For this review, take the finished solid that the model builds, in its own axes (mm). Round coordinates to 2 decimals unless told otherwise and drop trailing zeros. Order: outer loops, then holes, each group sorted by start corner. A loop starts at its lowest first (then second) coordinate and runs counter-clockwise, first axis right, second up. Notation, with made-up numbers: (74.25, 80) - (123.25, 80) arc R13 ccw to (123.25, 90) - close; hole circle Ø9 at (76, 50.5). An arc over 180 degrees is marked (long way). One line per question, with ' | ' between items.
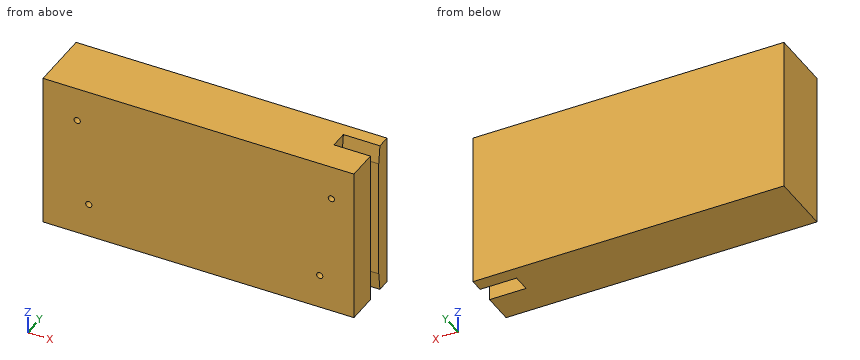
```python
from build123d import *

# Parameters (mm, degrees)
SCHIZZO2_W                   = 2000
SCHIZZO2_H                   = 1000
ESTRUSIONE_ESTRUSIONE1_DEPTH = 400
SVUOTA1_T                    = 40
SCHIZZO3_W                   = 320
SCHIZZO3_H                   = 545
ESTRUSIONE_ESTRUSIONE2_DEPTH = 285
SCHIZZO5_R                   = 20
TAGLIO_ESTRUSIONE1_DEPTH     = 40
SCHIZZO7_W                   = 235.156084519
SCHIZZO7_H                   = 1000
TAGLIO_ESTRUSIONE2_DEPTH     = 100
ESTRUSIONE_ESTRUSIONE4_DEPTH = 920
TAGLIO_ESTRUSIONE3_DEPTH     = 235.156084519


with BuildPart() as part:
    # Schizzo2 → Estrusione-Estrusione1 (new body)
    with BuildSketch(Plane(origin=(0, 0, 0), x_dir=(1, 0, 0), z_dir=(0, 1, 0))):
        Rectangle(SCHIZZO2_W, SCHIZZO2_H)
    extrude(amount=ESTRUSIONE_ESTRUSIONE1_DEPTH)

    # Svuota1 (no face opened: a closed hollow body)
    add(offset(amount=-SVUOTA1_T, mode=Mode.PRIVATE), mode=Mode.SUBTRACT)

    # Schizzo3 → Estrusione-Estrusione2 (add)
    with BuildSketch(Plane(origin=(0, 40, 0), x_dir=(1, 0, 0), z_dir=(0, 1, 0))):
        Rectangle(SCHIZZO3_W, SCHIZZO3_H)
    extrude(amount=ESTRUSIONE_ESTRUSIONE2_DEPTH)

    # Schizzo5 → Taglio-Estrusione1 (cut)
    with BuildSketch(Plane.XZ):
        with Locations(Location((-780, 280, 0), (0, 0, 270))):
            Circle(SCHIZZO5_R)
        with Locations(Location((780, -280, 0), (0, 0, 270))):
            Circle(SCHIZZO5_R)
        with Locations(Location((854.59, 280, 0), (0, 0, 270))):
            Circle(SCHIZZO5_R)
        with Locations(Location((-705.41, -280, 0), (0, 0, 270))):
            Circle(SCHIZZO5_R)
    extrude(amount=-TAGLIO_ESTRUSIONE1_DEPTH, mode=Mode.SUBTRACT)

    # Schizzo7 → Taglio-Estrusione2 (cut)
    with BuildSketch(Plane(origin=(0, 200, 0), x_dir=(1, 0, 0), z_dir=(0, 1, 0))):
        with Locations((882.421957741, 0)):
            Rectangle(SCHIZZO7_W, SCHIZZO7_H)
    extrude(amount=TAGLIO_ESTRUSIONE2_DEPTH, mode=Mode.SUBTRACT)

    # Schizzo8 → Estrusione-Estrusione4 (add)
    with BuildSketch(Plane.XY.offset(-460)):
        Polygon((960, 320), (724.843915481, 320), (724.843915481, 180), (960, 180), (960, 200), (764.843915481, 200), (764.843915481, 300), (960, 300), align=None)
    extrude(amount=ESTRUSIONE_ESTRUSIONE4_DEPTH)

    # Schizzo9 → Taglio-Estrusione3 (cut)
    with BuildSketch(Plane(origin=(1000, 0, 0), x_dir=(0, 0, -1), z_dir=(1, 0, 0))):
        Polygon((-500, 300), (-500, 314.392280451), (-382.784282115, 300), align=None)
        Polygon((382.784282115, 300), (500, 300), (500, 314.392280451), align=None)
    extrude(amount=-TAGLIO_ESTRUSIONE3_DEPTH, mode=Mode.SUBTRACT)


solid = part.part
```
(1) For probe 1 along X at (y, z) = (19, 280); probe 2 along X at (y, z) = (12, -280); probe 3 along Z at (x, y) = (83, 99.5), list the stretches that pass through material, from the lowest coordinate up. Write a range as [from, to].
Output values:
probe 1: [-1000, -800], [-760, 834.59], [874.59, 1000] | probe 2: [-1000, -725.41], [-685.41, 760], [800, 1000] | probe 3: [-500, -460], [-272.5, 272.5], [460, 500]
(2) We need section D-D on x = -780. State the section outline as (y, z) points, plus the area to 3 significant figures.
Output values:
outline: (0, -500) - (400, -500) - (400, 500) - (0, 500) - (0, 300) - (40, 300) - (40, 460) - (360, 460) - (360, -460) - (40, -460) - (40, 260) - (0, 260) - close | area: 104,000 mm^2
(3) We need section A-A on x = 854.59. State the section outline as (y, z) points, plus the area to 3 significant figures.
Output values:
outline: (0, -500) - (200, -500) - (200, 500) - (0, 500) - (0, 300) - (40, 300) - (40, 460) - (180, 460) - (180, -460) - (40, -460) - (40, 260) - (0, 260) - close; (300, -382.78) - (314.39, -500) - (400, -500) - (400, 500) - (314.39, 500) - (300, 382.78) - close; hole (320, -460) - (360, -460) - (360, 460) - (320, 460) - close | area: 131,000 mm^2
(4) Insertion check: pin 1 (6 mm diameter, centred on y = 271.5, z = 89, fed in from +X). The pin has a flat end and moves straight along its axis. Give the tip position at first contact, or say it passes through.
Output values:
pin 1: x = 764.84
(5) We need section B-B on x = 654. State the section outline as (y, z) points.
Output values:
outline: (0, -500) - (400, -500) - (400, 500) - (0, 500) - close; hole (40, -460) - (360, -460) - (360, 460) - (40, 460) - close
(6) We need section C-C on z = -225.5. State the section outline as (x, y) points, plus the area to 3 significant figures.
Output values:
outline: (-1000, 0) - (1000, 0) - (1000, 200) - (764.84, 200) - (764.84, 300) - (1000, 300) - (1000, 400) - (-1000, 400) - close; hole (-960, 40) - (-160, 40) - (-160, 325) - (160, 325) - (160, 40) - (960, 40) - (960, 180) - (724.84, 180) - (724.84, 320) - (960, 320) - (960, 360) - (-960, 360) - close | area: 286,000 mm^2
